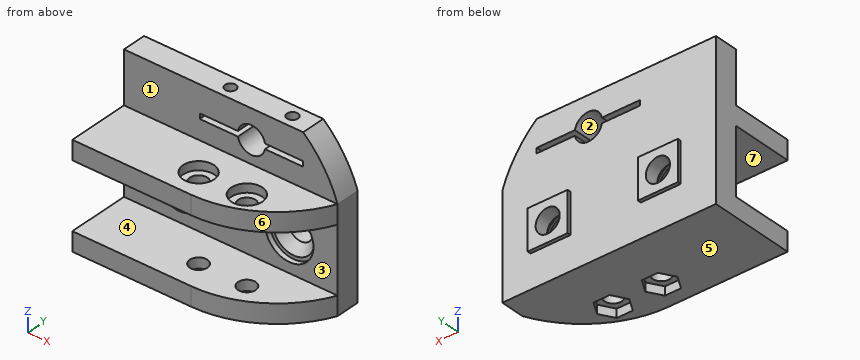
from build123d import *

# Parameters (mm, degrees)
SKETCH_W             = 62
SKETCH_H             = 25
PAD_DEPTH            = 15
SKETCH001_W          = 18
SKETCH001_H          = 19
POCKET_DEPTH         = 37.001
POCKET_DEPTH_BACK    = -25.001
SKETCH002_R          = 2.55
POCKET001_DEPTH      = 15.001
POCKET001_DEPTH_BACK = -15.001
SKETCH003_W          = 62
SKETCH003_H          = 7
PAD001_DEPTH         = 30
SKETCH004_R          = 4
POCKET002_DEPTH      = 12.501
SKETCH005_W          = 1
SKETCH005_H          = 11.6
PAD002_DEPTH         = 16.8
PAD002_DEPTH_BACK    = 26.8
SKETCH012_W          = 20.4
SKETCH012_H          = 1
POCKET003_DEPTH      = 11.6
SKETCH013_R          = 3.5
POCKET004_DEPTH      = 26.001
POCKET005_DEPTH      = 15.001
POCKET005_DEPTH_BACK = -30.001
POCKET006_DEPTH      = 13.501
SKETCH016_R          = 7
POCKET007_DEPTH      = 7
CHAMFER_SIZE         = 2.49
POCKET008_DEPTH      = 2.5
SKETCH019_R          = 4.5
POCKET009_DEPTH      = 2.5
SKETCH020_W          = 30
SKETCH020_H          = 1.5
POCKET010_DEPTH      = 8.001
SKETCH021_R          = 1.25
POCKET011_DEPTH      = 22
SKETCH022_R          = 1.6
POCKET012_DEPTH      = 8


with BuildPart() as part:
    # Sketch → Pad (new body, symmetric)
    with BuildSketch(Plane.XY):
        with Locations((-6, 0)):
            Rectangle(SKETCH_W, SKETCH_H)
    extrude(amount=PAD_DEPTH, both=True)

    # Sketch001 → Pocket (cut, two sides)
    with BuildSketch(Plane.YZ) as pocket_sk:
        with Locations((-3.5, 0)):
            Rectangle(SKETCH001_W, SKETCH001_H)
    extrude(amount=-POCKET_DEPTH, mode=Mode.SUBTRACT)
    extrude(pocket_sk.sketch, amount=-POCKET_DEPTH_BACK, mode=Mode.SUBTRACT)

    # Sketch002 → Pocket001 (cut, two sides)
    with BuildSketch(Plane.XY) as pocket001_sk:
        with Locations((-7, -4.5)):
            Circle(SKETCH002_R)
        with Locations((7, -4.5)):
            Circle(SKETCH002_R)
    extrude(amount=-POCKET001_DEPTH, mode=Mode.SUBTRACT)
    extrude(pocket001_sk.sketch, amount=-POCKET001_DEPTH_BACK, mode=Mode.SUBTRACT)

    # Sketch003 → Pad001 (join)
    with BuildSketch(Plane.XY):
        with Locations((-6, 9)):
            Rectangle(SKETCH003_W, SKETCH003_H)
    extrude(amount=PAD001_DEPTH)

    # Sketch004 → Pocket002 (cut, through all)
    with BuildSketch(Plane.XZ):
        with Locations((0, 21.5)):
            Circle(SKETCH004_R)
    extrude(amount=-POCKET002_DEPTH, mode=Mode.SUBTRACT)

    # Sketch005 → Pad002 (join, two sides)
    with BuildSketch(Plane.YZ) as pad002_sk:
        with Locations((13, 0.5)):
            Rectangle(SKETCH005_W, SKETCH005_H)
    extrude(amount=PAD002_DEPTH)
    extrude(pad002_sk.sketch, amount=-PAD002_DEPTH_BACK)

    # Sketch012 (on Face10 of Pad002) → Pocket003 (cut)
    with BuildSketch(Plane(origin=(0, 0, -5.3), x_dir=(1, 0, 0), z_dir=(0, 0, -1))):
        with Locations((-5, -13)):
            Rectangle(SKETCH012_W, SKETCH012_H)
    extrude(amount=-POCKET003_DEPTH, mode=Mode.SUBTRACT)

    # Sketch013 (on Face22 of Pocket003) → Pocket004 (cut, through all)
    with BuildSketch(Plane(origin=(0, 13.5, 0), x_dir=(-1, 0, 0), z_dir=(0, 1, 0))):
        with Locations((-11, 0.5)):
            Circle(SKETCH013_R)
        with Locations((21, 0.5)):
            Circle(SKETCH013_R)
    extrude(amount=-POCKET004_DEPTH, mode=Mode.SUBTRACT)

    # Sketch014 → Pocket005 (cut, two sides)
    with BuildSketch(Plane.XY) as pocket005_sk:
        with BuildLine():
            ThreePointArc((-2.495494, -12.5), (13.936206, -7.599812), (25, 5.5))
            Line((25, 5.5), (25, -12.5))
            Line((25, -12.5), (-2.495494, -12.5))
        make_face()
    extrude(amount=-POCKET005_DEPTH, mode=Mode.SUBTRACT)
    extrude(pocket005_sk.sketch, amount=-POCKET005_DEPTH_BACK, mode=Mode.SUBTRACT)

    # Sketch015 → Pocket006 (cut, through all)
    with BuildSketch(Plane.XZ):
        with BuildLine():
            ThreePointArc((25, 15), (20.982341, 23.154894), (15, 30))
            Line((25, 30), (15, 30))
            Line((25, 15), (25, 30))
        make_face()
    extrude(amount=-POCKET006_DEPTH, mode=Mode.SUBTRACT)

    # Sketch016 → Pocket007 (cut)
    with BuildSketch(Plane.XZ):
        with Locations((-21, 0.5)):
            Circle(SKETCH016_R)
        with Locations((11, 0.5)):
            Circle(SKETCH016_R)
    extrude(amount=-POCKET007_DEPTH, mode=Mode.SUBTRACT)

    # Chamfer
    chamfer_edges = [part.edges().sort_by_distance(p)[0] for p in [
        (-17.5, 7, 0.5),
        (14.5, 7, 0.5),
    ]]
    chamfer(chamfer_edges, length=CHAMFER_SIZE)

    # Sketch018 → Pocket008 (cut)
    with BuildSketch(Plane(origin=(0, 0, -15), x_dir=(1, 0, 0), z_dir=(0, 0, -1))):
        Polygon((-9.338269, 0.45), (-4.661731, 0.45), (-2.323463, 4.5), (-4.661731, 8.55), (-9.338269, 8.55), (-11.676537, 4.5), align=None)
        Polygon((9.338269, 0.45), (11.676537, 4.5), (9.338269, 8.55), (4.661731, 8.55), (2.323463, 4.5), (4.661731, 0.45), align=None)
    extrude(amount=-POCKET008_DEPTH, mode=Mode.SUBTRACT)

    # Sketch019 → Pocket009 (cut)
    with BuildSketch(Plane.XY.offset(15)):
        with Locations((-7, -4.5)):
            Circle(SKETCH019_R)
        with Locations((7, -4.5)):
            Circle(SKETCH019_R)
    extrude(amount=-POCKET009_DEPTH, mode=Mode.SUBTRACT)

    # Sketch020 (on Face40 of Pocket009) → Pocket010 (cut, through all)
    with BuildSketch(Plane.XZ.offset(-5.5)):
        with Locations((0, 21.5)):
            Rectangle(SKETCH020_W, SKETCH020_H)
    extrude(amount=-POCKET010_DEPTH, mode=Mode.SUBTRACT)

    # Sketch021 (on Face39 of Pocket010) → Pocket011 (cut)
    with BuildSketch(Plane.XY.offset(30)):
        with Locations((9, 9)):
            Circle(SKETCH021_R)
        with Locations((-9, 9)):
            Circle(SKETCH021_R)
    extrude(amount=-POCKET011_DEPTH, mode=Mode.SUBTRACT)

    # Sketch022 (on Face39 of Pocket011) → Pocket012 (cut)
    with BuildSketch(Plane.XY.offset(30)):
        with Locations((-9, 9)):
            Circle(SKETCH022_R)
        with Locations((9, 9)):
            Circle(SKETCH022_R)
    extrude(amount=-POCKET012_DEPTH, mode=Mode.SUBTRACT)


solid = part.part
For this review, take the finished solid that the model builds, in its own axes (mm). Face numbers are marked on the shaded views. A direction names the side the tool comes from. Round coordinates to 2 decimals unless told otherwise and drop trailing zeros. Order: outer loops, then holes, each group sorted by start corner. A loop starts at its lowest first (then second) coordinate and runs counter-clockwise, first axis right, second up. Notation, with made-up numbers: (35, 68.25) -> (42, 68.25) arc R18 ccw to (42, 99.25) -> close; hole circle Ø3 at (31, -2). An arc over 180 degrees is marked (long way). Write item = value, one per line. Start each with the question number.
1) Insertion check: pin 1 (8 mm diameter, centred on x = 7, y = -4.5, fed in from +Z); pin 2 (0.8 mm diameter, centred on x = 9.5, y = 8.5, fed in from +Z); pin 3 (3 mm diameter, centred on x = -9, y = 9, fed in from +Z). Each pin has a flat end and moves straight along its axis. Give the tip position at first contact, or say it passes through.
2) The part is to be moulded in two halves that separate along Z. For the marked faces 4, 5, 6 and 7, say which applies: +Z half, -Z half, draft (parallel to the pull), parting line (faces both ways), or undercut.
3) Take a section at D-D on x = 1.5. State the section outline as (y, z) points, plus the area to 3 significant figures.
4) To check wall thickness, follow line 1 (Y direction, x = 9, z = 17); line 2 (X direction, y = -2.5, z = -11); line 3 (Z direction, x = -8, y = -11). State the ranges of each line that lie inside material, in increasing order. Write a range as from..to.
5) Take a section at C-C on z = 0.5. Count the separate pieces of the cut face and the enclosed holes in it, plus the area to 3 significant figures.
6) Tool access review of the marked faces 1, 2 and 3: name each direction out of +Z, -Z, +X, -X, +Y, -Y from which nothing blocks a thin tool from reaching the whole face with its end or side.
7) Take a section at A-A on z = 19. State the section outline as (x, y) points, plus the area to 3 significant figures.
8) Take a section at B-B on x = -21. State the section outline as (y, z) points.
Verdict:
q1.pin_1 = 12.5
q1.pin_2 = 8
q1.pin_3 = 20.75
q2.face_4 = undercut
q2.face_5 = -Z half
q2.face_6 = draft
q2.face_7 = undercut
q3.outline = (-12.23, -15) -> (12.5, -15) -> (12.5, 17.79) -> (5.5, 17.79) -> (5.5, 15) -> (-12.23, 15) -> (-12.23, 9.5) -> (5.5, 9.5) -> (5.5, -9.5) -> (-12.23, -9.5) -> close; (5.5, 25.21) -> (12.5, 25.21) -> (12.5, 30) -> (5.5, 30) -> close
q3.area = 458 mm2
q4.line_1 = 5.5..7.75, 10.25..12.5
q4.line_2 = -37..-8.58, -5.42..5.42, 8.58..19.87
q4.line_3 = -15..-9.5, 9.5..15
q5.separate_pieces = 3
q5.enclosed_holes = 0
q5.area = 312 mm2
q6.face_1 = +Z, +X, -X, -Y
q6.face_2 = +Y, -Y
q6.face_3 = +X, -X, -Y
q7.outline = (-37, 5.5) -> (-3.12, 5.5) -> (-3.12, 12.5) -> (-37, 12.5) -> close; (3.12, 5.5) -> (23.36, 5.5) -> (23.36, 12.5) -> (3.12, 12.5) -> close; hole circle Ø2.5 at (-9, 9); hole circle Ø2.5 at (9, 9)
q7.area = 369 mm2
q8.outline = (-12.5, -15) -> (12.5, -15) -> (12.5, -5.3) -> (13.5, -5.3) -> (13.5, -3) -> (9.49, -3) -> (7, -5.49) -> (7, -6.5) -> (5.5, -6.5) -> (5.5, -9.5) -> (-12.5, -9.5) -> close; (-12.5, 9.5) -> (5.5, 9.5) -> (5.5, 7.5) -> (7, 7.5) -> (7, 6.49) -> (9.49, 4) -> (13.5, 4) -> (13.5, 6.3) -> (12.5, 6.3) -> (12.5, 30) -> (5.5, 30) -> (5.5, 15) -> (-12.5, 15) -> close
